For this review, take the finished solid that the model builds, in its own axes (mm). Face numbers are marked on the shaded views. A direction names the side the tool comes from. Coordinates: 2 decimals unless noted, no trailing zeros. Loops run counter-clockwise (first coordinate to the right, second up) from the corner with the lowest first, then second, coordinate; pieces in that order, holes last. Notation, with made-up numbers: M -16.75,56 L 27.25,56 A20 ccw 27.25,87 Z; hole C 26,34 d1. An arc over 180 degrees is marked long. Write item = value, one per line.
Autodesk Fusion 360 part; units mm, degrees
sketch "Esquisse1" plane through (0, 0, 0) normal (0, 0, 1) x (1, 0, 0)
  line L0 (50, 0) -> (0, 0)
  line L1 (0, 0) -> (0, 72)
  line L2 (0, 72) -> (50, 72)
  line L3 (50, 72) -> (50, 0)
  line L4 (42, 64) -> (8, 64)
  line L5 (8, 64) -> (8, 8)
  line L6 (8, 8) -> (42, 8)
  line L7 (42, 8) -> (42, 64)
  dimension "d3" = 72
  dimension "d4" = 50
  dimension "d26" = 8
  dimension "d27" = 8
  dimension "d28" = 8
  dimension "d29" = 8
extrude "Extrusion1" add sketch "Esquisse1" along normal blind 9
sketch "Esquisse2" plane through (0, 0, 0) normal (0, -1, 0) x (1, 0, 0)
  line L0 (0, 0) -> (50, 0)
  line L1 (50, 9) -> (0, 9)
  line L2 (0, 9) -> (0, 0)
  line L3 (-5.7525, 4.5) -> (21.5406, 4.5) construction
  circle A0 centre (5, 4.5) radius 2.175
  circle A1 centre (12, 4.5) radius 2.175
  line L4 (50, 0) -> (50, 9)
  dimension "d7" = 4.35
  dimension "d8" = 7
  dimension "d9" = 4.5
  dimension "d10" = 5
extrude "Extrusion2" cut sketch "Esquisse2" against normal blind 8 contours A0 | A1
sketch "Esquisse3" plane through (0, 72, 0) normal (0, 1, 0) x (-1, 0, 0)
  line L0 (-50, 0) -> (0, 0)
  line L1 (0, 0) -> (0, 9)
  line L2 (0, 9) -> (-50, 9)
  line L3 (5.6122, 4.5) -> (-27.7174, 4.5) construction
  circle A0 centre (-12, 4.5) radius 2.175
  circle A1 centre (-5, 4.5) radius 2.175
  line L4 (-50, 9) -> (-50, 0)
  dimension "d13" = 4.5
  dimension "d14" = 7
  dimension "d15" = 5
  dimension "d16" = 4.35
extrude "Extrusion3" cut sketch "Esquisse3" against normal blind 8 contours A0 | A1
sketch "Esquisse4" plane through (0, 0, 0) normal (-1, 0, 0) x (0, 0, 1)
  line L0 (0, 72) -> (0, 0)
  line L1 (0, 0) -> (9, 0)
  line L2 (9, 0) -> (9, 72)
  line L3 (9, 72) -> (0, 72)
  line L4 (4.5, 76) -> (4.5, -2) construction
  circle A0 centre (4.5, 12.5) radius 2.175
  circle A1 centre (4.5, 59.5) radius 2.175
  circle A2 centre (4.5, 36) radius 2.175
  dimension "d19" = 4.35
  dimension "d20" = 12.5
  dimension "d21" = 12.5
  dimension "d22" = 23.5
  dimension "d25" = 4.5
extrude "Extrusion4" cut sketch "Esquisse4" against normal blind 8 contours A0 | A1 | A2
chamfer "Chanfrein1" distance 1 angle 45 4 edges at (25, 0, 9) (25, 72, 9) (25, 72, 0) (25, 0, 0)
equation "d21 = d20"
equation "d22 = ( 47 / 2 ) * 1 mm"
equation "d27 = d26"
equation "d28 = d26"
equation "d29 = d26"
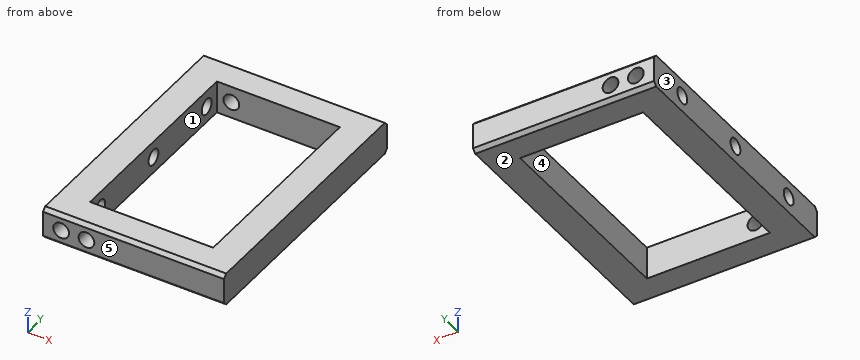
Q1. Add section B-B (x = 12). Write out the cut boundary in (y, z) (3 decimals).
Solved:
outline = M 0,1 L 1,0 L 8,0 L 8,2.325 L 0,2.325 Z; M 0,6.675 L 8,6.675 L 8,9 L 1,9 L 0,8 Z; M 64,0 L 71,0 L 72,1 L 72,2.325 L 64,2.325 Z; M 64,6.675 L 72,6.675 L 72,8 L 71,9 L 64,9 Z
Q2. Draft analysis for pull direction X (two halves, no side actions). For the marked faces 1, 2 and 3, state which applies: +X half, -X half, draft (parallel to the pull), parting line (faces both ways), or undercut.
Solved:
face_1 = undercut
face_2 = draft
face_3 = -X half
Q3. Add section D-D (x = 5). Write out the cut boundary in (y, z) (3 decimals).
Solved:
outline = M 0,1 L 1,0 L 71,0 L 72,1 L 72,2.325 L 64,2.325 L 64,6.675 L 72,6.675 L 72,8 L 71,9 L 1,9 L 0,8 L 0,6.675 L 8,6.675 L 8,2.325 L 0,2.325 Z; hole C 12.5,4.5 d4.35; hole C 36,4.5 d4.35; hole C 59.5,4.5 d4.35
Q4. Add section C-C (y = 12.5). Write out the cut boundary in (x, z) (3 decimals), and give its area (3 significant figures).
Solved:
outline = M 0,0 L 8,0 L 8,2.325 L 0,2.325 Z; M 0,6.675 L 8,6.675 L 8,9 L 0,9 Z; M 42,0 L 50,0 L 50,9 L 42,9 Z
area = 109 mm²
Q5. For line 1 along X through (y, z) = (38, 2.25); line 2 along Y through (x, z) = (28, 5.25); line 3 along Z through (x, y) = (5, 2.5) (3 decimals), list the stretches that pass through material, from the lowest coordinate up.
Solved:
line_1 = 0 to 8, 42 to 50
line_2 = 0 to 8, 64 to 72
line_3 = 0 to 2.325, 6.675 to 9
Q6. Add section A-A (y = 47). Write out the cut boundary in (x, z).
Solved:
outline = M 0,0 L 8,0 L 8,9 L 0,9 Z; M 42,0 L 50,0 L 50,9 L 42,9 Z
Q7. Machinability: for the marked faces 4 and 5, which of the approach directions +Z, -Z, +X, -X, +Y, -Y give a long, thin tool a straight path to every point of the face, cutting with its end or side? Answer none if there is none.
Solved:
face_4 = +Z, -Z
face_5 = +Z, -Z, +X, -X, -Y
